Check sheet for the modelled part. Datum: model origin and axes. Units: mm. Give positions to 0.01 mm unless a question says otherwise; leave off trailing zeros. Loops run counter-clockwise (first coordinate to the right, second up) from the corner with the lowest first, then second, coordinate; pieces in that order, holes last. Notation, with made-up numbers: (70, 72) - (101, 72) arc R6 ccw to (101, 81) - close; hole circle Ø10 at (-21, 87.5). An arc over 180 degrees is marked (long way). Use CSV: the item, a comma, the result in double quotes.
from build123d import *

# Parameters (mm, degrees)
SKETCH1_R           = 1.5
BOSS_EXTRUDE1_DEPTH = 1.5
CUT_EXTRUDE1_DEPTH  = 1.5


with BuildPart() as part:
    # Sketch1 → Boss-Extrude1 (new body)
    with BuildSketch(Plane(origin=(0, 0, 0), x_dir=(1, 0, 0), z_dir=(0, 1, 0))):
        Polygon((0, 93.25), (-24.863047384, 90.636788418), (-24.863047384, 70.636788418), (-38.863047384, 46.388077112), (-24.863047384, 22.139365806), (-24.863047384, -22.139365806), (-38.863047384, -46.388077112), (-24.863047384, -70.636788418), (-24.863047384, -90.636788418), (0, -93.25), (24.863047384, -90.636788418), (24.863047384, -70.636788418), (38.863047384, -46.388077112), (24.863047384, -22.139365806), (24.863047384, 22.139365806), (38.863047384, 46.388077112), (24.863047384, 70.636788418), (24.863047384, 90.636788418), align=None)
        with Locations(Location((0, 50.25, 0), (0, 0, 270))):
            Circle(SKETCH1_R, mode=Mode.SUBTRACT)
        with Locations(Location((-9, 45.25, 0), (0, 0, 270))):
            Circle(SKETCH1_R, mode=Mode.SUBTRACT)
        with Locations(Location((-15, 55.25, 0), (0, 0, 270))):
            Circle(SKETCH1_R, mode=Mode.SUBTRACT)
        with Locations(Location((-9, 65.25, 0), (0, 0, 270))):
            Circle(SKETCH1_R, mode=Mode.SUBTRACT)
        with Locations(Location((9, 45.25, 0), (0, 0, 90))):
            Circle(SKETCH1_R, mode=Mode.SUBTRACT)
        with Locations(Location((9, 65.25, 0), (0, 0, 90))):
            Circle(SKETCH1_R, mode=Mode.SUBTRACT)
        with Locations(Location((15, 55.25, 0), (0, 0, 90))):
            Circle(SKETCH1_R, mode=Mode.SUBTRACT)
        with Locations(Location((-15.25, 15.25, 0), (0, 0, 270))):
            Circle(SKETCH1_R, mode=Mode.SUBTRACT)
        with Locations(Location((15.25, 15.25, 0), (0, 0, 90))):
            Circle(SKETCH1_R, mode=Mode.SUBTRACT)
        with Locations(Location((-32.863047384, 46.388077112, 0), (0, 0, 270))):
            Circle(SKETCH1_R, mode=Mode.SUBTRACT)
        with Locations(Location((-17.363047384, 82.75, 0), (0, 0, 270))):
            Circle(SKETCH1_R, mode=Mode.SUBTRACT)
        with Locations(Location((32.863047384, 46.388077112, 0), (0, 0, 90))):
            Circle(SKETCH1_R, mode=Mode.SUBTRACT)
        with Locations(Location((17.363047384, 82.75, 0), (0, 0, 90))):
            Circle(SKETCH1_R, mode=Mode.SUBTRACT)
        with Locations(Location((-15.25, -15.25, 0), (0, 0, 90))):
            Circle(SKETCH1_R, mode=Mode.SUBTRACT)
        with Locations(Location((15.25, -15.25, 0), (0, 0, 270))):
            Circle(SKETCH1_R, mode=Mode.SUBTRACT)
        with Locations(Location((32.863047384, -46.388077112, 0), (0, 0, 270))):
            Circle(SKETCH1_R, mode=Mode.SUBTRACT)
        with Locations(Location((9, -45.25, 0), (0, 0, 270))):
            Circle(SKETCH1_R, mode=Mode.SUBTRACT)
        with Locations(Location((-32.863047384, -46.388077112, 0), (0, 0, 90))):
            Circle(SKETCH1_R, mode=Mode.SUBTRACT)
        with Locations(Location((-9, -45.25, 0), (0, 0, 90))):
            Circle(SKETCH1_R, mode=Mode.SUBTRACT)
        with Locations(Location((15, -55.25, 0), (0, 0, 270))):
            Circle(SKETCH1_R, mode=Mode.SUBTRACT)
        with Locations(Location((0, -50.25, 0), (0, 0, 90))):
            Circle(SKETCH1_R, mode=Mode.SUBTRACT)
        with Locations(Location((-15, -55.25, 0), (0, 0, 90))):
            Circle(SKETCH1_R, mode=Mode.SUBTRACT)
        with Locations(Location((-9, -65.25, 0), (0, 0, 90))):
            Circle(SKETCH1_R, mode=Mode.SUBTRACT)
        with Locations(Location((9, -65.25, 0), (0, 0, 270))):
            Circle(SKETCH1_R, mode=Mode.SUBTRACT)
        with Locations(Location((17.363047384, -82.75, 0), (0, 0, 270))):
            Circle(SKETCH1_R, mode=Mode.SUBTRACT)
        with Locations(Location((-17.363047384, -82.75, 0), (0, 0, 90))):
            Circle(SKETCH1_R, mode=Mode.SUBTRACT)
        with BuildLine():
            Line((-3, 5.25), (3, 5.25))
            ThreePointArc((3, 5.25), (4.414213562, 5.835786438), (5, 7.25))
            Line((5, 7.25), (5, 23.25))
            ThreePointArc((5, 23.25), (4.414213562, 24.664213562), (3, 25.25))
            Line((3, 25.25), (-3, 25.25))
            ThreePointArc((-3, 25.25), (-4.414213562, 24.664213562), (-5, 23.25))
            Line((-5, 23.25), (-5, 7.25))
            ThreePointArc((-5, 7.25), (-4.414213562, 5.835786438), (-3, 5.25))
        make_face(mode=Mode.SUBTRACT)
        with BuildLine():
            Line((-10.2, 6.25), (-10.2, 24.25))
            ThreePointArc((-10.2, 24.25), (-9.2, 25.25), (-8.2, 24.25))
            Line((-8.2, 24.25), (-8.2, 6.25))
            ThreePointArc((-8.2, 6.25), (-9.2, 5.25), (-10.2, 6.25))
        make_face(mode=Mode.SUBTRACT)
        with BuildLine():
            Line((10.2, 6.25), (10.2, 24.25))
            ThreePointArc((10.2, 24.25), (9.2, 25.25), (8.2, 24.25))
            Line((8.2, 24.25), (8.2, 6.25))
            ThreePointArc((8.2, 6.25), (9.2, 5.25), (10.2, 6.25))
        make_face(mode=Mode.SUBTRACT)
        with BuildLine():
            Line((5, -7.25), (5, -23.25))
            ThreePointArc((5, -23.25), (4.414213562, -24.664213562), (3, -25.25))
            Line((3, -25.25), (-3, -25.25))
            ThreePointArc((-3, -25.25), (-4.414213562, -24.664213562), (-5, -23.25))
            Line((-5, -23.25), (-5, -7.25))
            ThreePointArc((-5, -7.25), (-4.414213562, -5.835786438), (-3, -5.25))
            Line((-3, -5.25), (3, -5.25))
            ThreePointArc((3, -5.25), (4.414213562, -5.835786438), (5, -7.25))
        make_face(mode=Mode.SUBTRACT)
        with BuildLine():
            Line((10.2, -6.25), (10.2, -24.25))
            ThreePointArc((10.2, -24.25), (9.2, -25.25), (8.2, -24.25))
            Line((8.2, -24.25), (8.2, -6.25))
            ThreePointArc((8.2, -6.25), (9.2, -5.25), (10.2, -6.25))
        make_face(mode=Mode.SUBTRACT)
        with BuildLine():
            Line((-10.2, -6.25), (-10.2, -24.25))
            ThreePointArc((-10.2, -24.25), (-9.2, -25.25), (-8.2, -24.25))
            Line((-8.2, -24.25), (-8.2, -6.25))
            ThreePointArc((-8.2, -6.25), (-9.2, -5.25), (-10.2, -6.25))
        make_face(mode=Mode.SUBTRACT)
    extrude(amount=BOSS_EXTRUDE1_DEPTH)

    # Sketch2 → Cut-Extrude1 (cut)
    with BuildSketch(Plane(origin=(0, 1.5, 0), x_dir=(1, 0, 0), z_dir=(0, 1, 0))):
        with BuildLine():
            Line((-8, 79.5), (8, 79.5))
            ThreePointArc((8, 79.5), (9.414213562, 80.085786438), (10, 81.5))
            Line((10, 81.5), (10, 84))
            ThreePointArc((10, 84), (9.267766953, 85.767766953), (7.5, 86.5))
            Line((7.5, 86.5), (-7.5, 86.5))
            ThreePointArc((-7.5, 86.5), (-9.267766953, 85.767766953), (-10, 84))
            Line((-10, 84), (-10, 81.5))
            ThreePointArc((-10, 81.5), (-9.414213562, 80.085786438), (-8, 79.5))
        make_face()
        with BuildLine():
            Line((10, -81.5), (10, -84))
            ThreePointArc((10, -84), (9.267766953, -85.767766953), (7.5, -86.5))
            Line((7.5, -86.5), (-7.5, -86.5))
            ThreePointArc((-7.5, -86.5), (-9.267766953, -85.767766953), (-10, -84))
            Line((-10, -84), (-10, -81.5))
            ThreePointArc((-10, -81.5), (-9.414213562, -80.085786438), (-8, -79.5))
            Line((-8, -79.5), (8, -79.5))
            ThreePointArc((8, -79.5), (9.414213562, -80.085786438), (10, -81.5))
        make_face()
    extrude(amount=-CUT_EXTRUDE1_DEPTH, mode=Mode.SUBTRACT)


solid = part.part
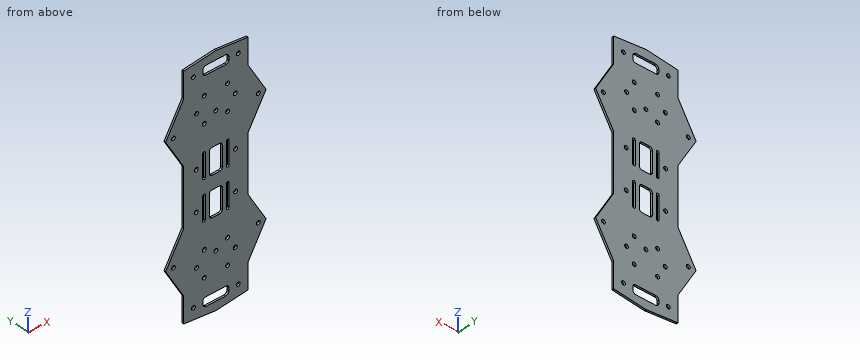
1. Sectioned sample at B-B, the plane y = 0.9. State how many separate pieces and enclosed holes the cut face has, and give its area (3 significant figures).
Completed:
separate pieces,"1"
enclosed holes,"34"
area,"9,500 mm²"
2. Sectioned sample at A-A, the plane z = 2.5. Record the boundary of the cut face in (x, y).
Completed:
outline,"(-24.86, 0) - (24.86, 0) - (24.86, 1.5) - (-24.86, 1.5) - close"
3. Scan lines: line 1 along X through (y, z) = (1.2, -20.5); line 2 along X through (y, z) = (0.6, -82.75); line 3 along Z through (x, y) = (3, 0.8). Record each from-to range of solid material in increasing order.
Completed:
line 1,"x = -24.86 to -10.2, -8.2 to -5, 5 to 8.2, 10.2 to 24.86"
line 2,"x = -24.86 to -18.86, -15.86 to -10, 10 to 15.86, 18.86 to 24.86"
line 3,"z = -92.93 to -86.5, -79.5 to -25.25, -5.25 to 5.25, 25.25 to 79.5, 86.5 to 92.93"
4. Sectioned sample at C-C, the plane x = -23. Record the boundary of the cut face in (y, z).
Completed:
outline,"(0, -90.83) - (1.5, -90.83) - (1.5, 90.83) - (0, 90.83) - close"
5. Go/stop test with flat-tipped pins: pin 1 Ø2.5 at (x, z) = (15.25, -15.25) entering from -Y; pin 2 Ø0.8 at (y, z) = (0.5, -82.5) entering from +X; pin 3 Ø0.8 at (y, z) = (1, -11) entering from -X. Record where each tip stops, or that it passes through.
Completed:
pin 1,"passes through"
pin 2,"stops at x = 24.86"
pin 3,"stops at x = -24.86"
